```python
from build123d import *

# Parameters (mm, degrees)
SKETCH1_R           = 50
BOSS_EXTRUDE1_DEPTH = 5
SKETCH2_R           = 1.9
CUT_EXTRUDE1_DEPTH  = 6
CIRPATTERN1_COUNT   = 4
SKETCH3_R           = 17.5
CUT_EXTRUDE2_DEPTH  = 6
CIRPATTERN2_COUNT   = 4
SKETCH4_R           = 8
SKETCH4_R_2         = 3
SKETCH4_R_3         = 2.5
SKETCH4_R_4         = 2
CUT_EXTRUDE3_DEPTH  = 6
CIRPATTERN3_COUNT   = 4


with BuildPart() as part:
    # Sketch1 → Boss-Extrude1 (new body)
    with BuildSketch(Plane.XY):
        Circle(SKETCH1_R)
    extrude(amount=BOSS_EXTRUDE1_DEPTH)

    # Sketch2 → Cut-Extrude1 (cut, through all)
    with BuildSketch(Plane(origin=(0, 0, 0), x_dir=(-1, 0, 0), z_dir=(0, 0, -1))):
        with Locations((-5.656854249, 5.656854249)):
            Circle(SKETCH2_R)
    cut_extrude1 = extrude(amount=-CUT_EXTRUDE1_DEPTH, mode=Mode.SUBTRACT)

    # CirPattern1: Cut-Extrude1 ×4 about axis
    cirpattern1_axis = Axis((0, 0, 0), (0, 0, 1))
    for i in range(1, CIRPATTERN1_COUNT):
        add(cut_extrude1.rotate(cirpattern1_axis, i * 360 / CIRPATTERN1_COUNT), mode=Mode.SUBTRACT)

    # Sketch3 → Cut-Extrude2 (cut, through all)
    with BuildSketch(Plane(origin=(0, 0, 0), x_dir=(-1, 0, 0), z_dir=(0, 0, -1))):
        with Locations((0, 30)):
            Circle(SKETCH3_R)
    cut_extrude2 = extrude(amount=-CUT_EXTRUDE2_DEPTH, mode=Mode.SUBTRACT)

    # CirPattern2: Cut-Extrude2 ×4 about axis
    cirpattern2_axis = Axis((0, 0, 0), (0, 0, 1))
    for i in range(1, CIRPATTERN2_COUNT):
        add(cut_extrude2.rotate(cirpattern2_axis, i * 360 / CIRPATTERN2_COUNT), mode=Mode.SUBTRACT)

    # Sketch4 → Cut-Extrude3 (cut, through all)
    with BuildSketch(Plane(origin=(0, 0, 0), x_dir=(-1, 0, 0), z_dir=(0, 0, -1))):
        with Locations((-28.284271247, 28.284271247)):
            Circle(SKETCH4_R)
        with Locations((-18.686291501, 18.686291501)):
            Circle(SKETCH4_R_2)
        with Locations((-13.736544033, 13.736544033)):
            Circle(SKETCH4_R_3)
        with Locations((-9.493903346, 9.493903346)):
            Circle(SKETCH4_R_4)
        with Locations((-20.231783609, 40.939603832)):
            Circle(SKETCH4_R_4)
        with Locations((-40.939603832, 20.231783609)):
            Circle(SKETCH4_R_4)
    cut_extrude3 = extrude(amount=-CUT_EXTRUDE3_DEPTH, mode=Mode.SUBTRACT)

    # CirPattern3: Cut-Extrude3 ×4 about axis
    cirpattern3_axis = Axis((0, 0, 0), (0, 0, 1))
    for i in range(1, CIRPATTERN3_COUNT):
        add(cut_extrude3.rotate(cirpattern3_axis, i * 360 / CIRPATTERN3_COUNT), mode=Mode.SUBTRACT)


solid = part.part
```
Here's how the part is built. I have some questions about the finished solid (model axes, mm). Coordinates: 2 decimals unless noted, no trailing zeros. Order: outer loops, then holes, each group sorted by start corner. A loop starts at its lowest first (then second) coordinate and runs counter-clockwise, first axis right, second up. Notation, with made-up numbers: (61.25, -35) -> (107.25, -35) arc R33 cw to (107.25, 3) -> close; hole circle Ø6 at (34.5, 54.5). An arc over 180 degrees is marked (long way). Return JSON: item names as keys, results as strings.
1) If I drill on probe 1 along Y at (x, z) = (1.5, 1.95); probe 2 along Y at (x, z) = (-31.5, 0.6); probe 3 along Y at (x, z) = (0, 2.1), over which ranges is the centre line in solid material (lowest first)?
Conclusion:
{"probe 1": "y = -49.98 to -47.44, -12.56 to 12.56, 47.44 to 49.98", "probe 2": "y = -38.83 to -35.61, -20.96 to -17.44, 17.44 to 20.96, 35.61 to 38.83", "probe 3": "y = -50 to -47.5, -12.5 to 12.5, 47.5 to 50"}
2) Thinking about a two-plate mould opening in X: for faces 1 (the cylindrical face through (11.477, -9.754, 2.465)), 2 (the flat face through (0, -3, 0)), 3 (the cylindrical face through (47.69, 15.02, 2.46)), which applies, +X half, -X half, draft (parallel to the pull), parting line (faces both ways), or undercut?
Conclusion:
{"face 1": "undercut", "face 2": "draft", "face 3": "parting line"}
3) If we section it at C-C on x = -30: List the corners of the cut face in (y, z) for me.
Conclusion:
{"outline": "(-40, 0) -> (-36.1, 0) -> (-36.1, 5) -> (-40, 5) -> close; (-20.47, 0) -> (-17.5, 0) -> (-17.5, 5) -> (-20.47, 5) -> close; (17.5, 0) -> (20.47, 0) -> (20.47, 5) -> (17.5, 5) -> close; (36.1, 0) -> (40, 0) -> (40, 5) -> (36.1, 5) -> close"}
4) If we section it at D-D on z = 2.25: State how many separate pieces and enclosed holes the cut face has, plus the area to 3 significant figures.
Conclusion:
{"separate pieces": "1", "enclosed holes": "32", "area": "2,810 mm²"}
5) I'm going to push flat-ended pins straight in: P1, Ø3.5, axis at x = 5.66, y = -5.66, coming from the +Z side; P2, Ø2, axis at x = -18, z = 1, coming from the +Y side; P3, Ø2, axis at y = -35, z = 3, coming from the +X side. Where does each tip first touch, or does it pass through?
Conclusion:
{"P1": "passes through", "P2": "stops at y = 47.02", "P3": "stops at x = 36.66"}
6) If we section it at A-A on x = 0: List the corners of the cut face in (y, z) for me, plus the area to 3 significant figures.
Conclusion:
{"outline": "(-50, 0) -> (-47.5, 0) -> (-47.5, 5) -> (-50, 5) -> close; (-12.5, 0) -> (12.5, 0) -> (12.5, 5) -> (-12.5, 5) -> close; (47.5, 0) -> (50, 0) -> (50, 5) -> (47.5, 5) -> close", "area": "150 mm²"}
